from build123d import *

# Parameters (mm, degrees)
F2_R     = 19.75
F2_R_2   = 17.75
F3_DEPTH = 10
F4_DEPTH = 7
F5_R     = 3


with BuildPart() as f3:
    # F2 (on Top) → F3 (new body)
    with BuildSketch(Plane.XY):
        Circle(F2_R)
        Circle(F2_R_2, mode=Mode.SUBTRACT)
        Circle(F2_R_2)
    extrude(amount=F3_DEPTH)

    # F2 (on Top) → F4 (cut)
    with BuildSketch(Plane.XY):
        Circle(F2_R_2)
    extrude(amount=F4_DEPTH, mode=Mode.SUBTRACT)

    # F5
    f5_edges = [f3.edges().sort_by_distance(p)[0] for p in [
        (-19.75, 0, 10),
    ]]
    fillet(f5_edges, radius=F5_R)


solid = f3.part
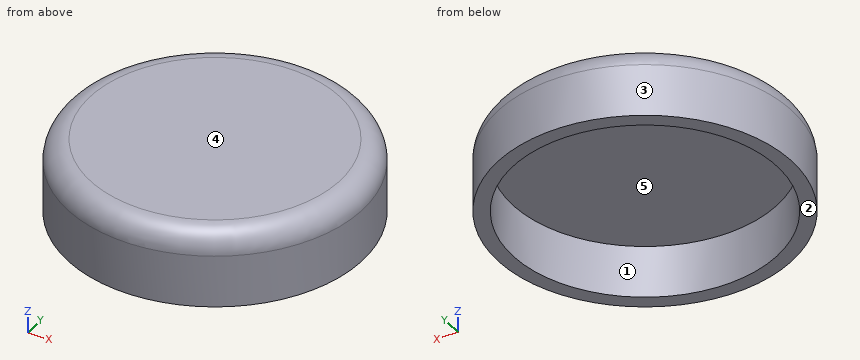
Here's how the part is built. I have some questions about the finished solid (model axes, mm). Face numbers are marked on the shaded views. A direction names the side the tool comes from. Give positions to 0.01 mm unless a question says otherwise; leave off trailing zeros. Loops run counter-clockwise (first coordinate to the right, second up) from the corner with the lowest first, then second, coordinate; pieces in that order, holes last. Notation, with made-up numbers: (-15.75, -33.5) -> (29.25, -33.5) arc R21 ccw to (29.25, 3.5) -> close; hole circle Ø6 at (-21.5, 18.5). An arc over 180 degrees is marked (long way). Answer as a JSON object with one key per item and string values. Group by question number.
Item 1: I need wall thicknesses on L1, parallel to Y at x = 0, z = 4.5; L2, parallel to Z at x = -9, y = 0.5; L3, parallel to Y at x = -15, z = 4. Which ranges of each line are inside material? Lowest first, please.
Item 2: Imagine slicing it at C-C on z = 2.75. Write out the boundary of the cut face in (x, y).
Item 3: Will these pins go through, and if not, where does the flat tip stop? pin 1 (10.5 mm diameter, centred on x = -3.5, y = 1, fed in from -Z); pin 2 (3 mm diameter, centred on y = 9.5, z = 6.5, fed in from -X); pin 3 (6 mm diameter, centred on x = 13, y = -12, fed in from +Z); pin 4 (1 mm diameter, centred on x = -9.5, z = 7, fed in from +Y).
Item 4: On a 3-axis mill with a long thin cutter (end or side, diameter ignored), from which of +Z, -Z, +X, -X, +Y, -Y can I reach the whole of each face in a straight line? I mean the marked faces 1 and 2. Say none if no direction works.
Item 5: Thinking about a two-plate mould opening in Y: for the marked faces 3, 4 and 5, which applies, pulls with the +Y half, pulls with the -Y half, needs draft (parallel to the pull), parting line crosses it, or undercut?
Item 6: Imagine slicing it at A-A on y = 0. Write out the boundary of the cut face in (x, z), then the cut area to 3 significant figures.
Answer list:
{
 "1": {"L1": "y = -19.75 to -17.75, 17.75 to 19.75", "L2": "z = 7 to 10", "L3": "y = -12.85 to -9.49, 9.49 to 12.85"},
 "2": {"outline": "circle Ø39.5 at (0, 0); hole circle Ø35.5 at (0, 0)"},
 "3": {"pin 1": "stops at z = 7", "pin 2": "stops at x = -18.06", "pin 3": "stops at z = 10", "pin 4": "stops at y = 17.58"},
 "4": {"face 1": "-Z", "face 2": "-Z, +X, -X, +Y, -Y"},
 "5": {"face 3": "parting line crosses it", "face 4": "needs draft", "face 5": "undercut"},
 "6": {"outline": "(-19.75, 0) -> (-17.75, 0) -> (-17.75, 7) -> (17.75, 7) -> (17.75, 0) -> (19.75, 0) -> (19.75, 7) arc R3 ccw to (16.75, 10) -> (-16.75, 10) arc R3 ccw to (-19.75, 7) -> close", "area": "143 mm2"}
}
